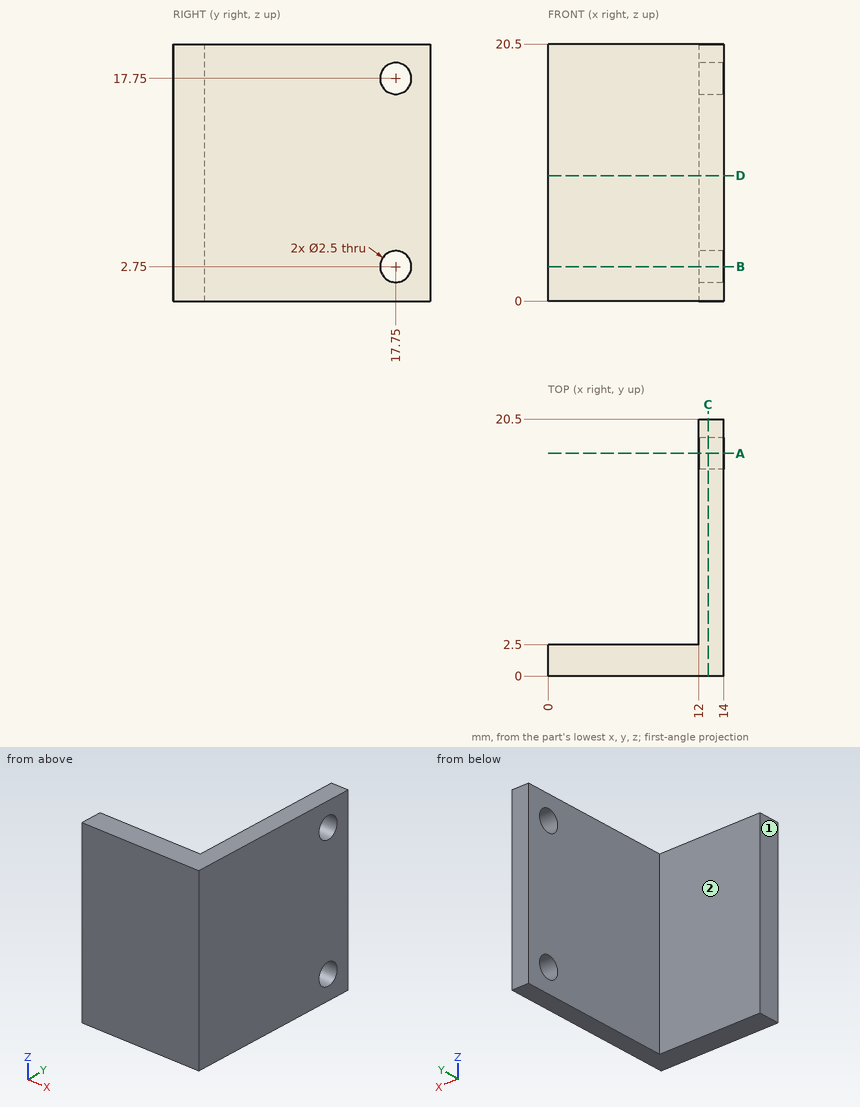
Answer from the drawing. Dimensions are ordinates in mm from the lowest x, y and z of the part. A direction names the side the tool comes from. Give positions to 0.01 mm unless a question says otherwise; leave off trailing zeros. Order: outer loops, then holes, each group sorted by start corner. A loop starts at its lowest first (then second) coordinate and runs counter-clockwise, first axis right, second up. Notation, with made-up numbers: (27.25, 24) -> (64.25, 24) arc R13 ccw to (64.25, 46) -> close; hole circle Ø7 at (61, 80). An arc over 180 degrees is marked (long way). One line per item, written item: value. Start each with the question number.
(1) The part is cut by section C-C (x = 12.75). Determine the outline of the cut face in (y, z), and give its area (3 significant figures).
(2) The part is cut by section B-B (z = 2.75). Determine the outline of the cut face in (x, y).
(3) Straight lines are drawn through the part: L1, parallel to Y at x = 12.55, z = 2.75; L2, parallel to Y at x = 2, z = 11.75; L3, parallel to X at y = 6.75, z = 9. For each, find the intervals that lie inside material, in ascending order.
(4) The part is cut by section D-D (z = 10). Determine the outline of the cut face in (x, y), and give its area (3 significant figures).
(5) A tool of negligible diameter and unlimited length cuts with its end or side. For the marked faces 1 and 2, from which of +Z, -Z, +X, -X, +Y, -Y can it reach the whole face along a straight path? Write none if from no direction.
(6) The part is cut by section A-A (y = 17.75). Determine the outline of the cut face in (x, z).
(7) Flat-ended cylindrical pins translate along their axes: P1, Ø4, axis at x = 11.5, y = 16.5, coming from the +Z side; P2, Ø1.5, axis at x = 2, z = 9.5, coming from the +Y side; P3, Ø8, axis at y = 13.5, z = 8.5, coming from the -X side; P4, Ø2, axis at y = 17.75, z = 2.75, coming from the +X side. Find the tip coordinate at first contact, or state that the pin passes through.
Taken from the geometry:
1. outline: (0, 0) -> (20.5, 0) -> (20.5, 20.5) -> (0, 20.5) -> close; hole circle Ø2.5 at (17.75, 2.75); hole circle Ø2.5 at (17.75, 17.75)
1. area: 410 mm^2
2. outline: (0, 0) -> (14, 0) -> (14, 16.5) -> (12, 16.5) -> (12, 2.5) -> (0, 2.5) -> close; (12, 19) -> (14, 19) -> (14, 20.5) -> (12, 20.5) -> close
3. L1: 0 to 16.5, 19 to 20.5
3. L2: 0 to 2.5
3. L3: 12 to 14
4. outline: (0, 0) -> (14, 0) -> (14, 20.5) -> (12, 20.5) -> (12, 2.5) -> (0, 2.5) -> close
4. area: 71.0 mm^2
5. face 1: +Z, -Z, -X, +Y, -Y
5. face 2: +Z, -Z, -X, +Y
6. outline: (12, 0) -> (14, 0) -> (14, 1.5) -> (12, 1.5) -> close; (12, 4) -> (14, 4) -> (14, 16.5) -> (12, 16.5) -> close; (12, 19) -> (14, 19) -> (14, 20.5) -> (12, 20.5) -> close
7. P1: z = 20.5
7. P2: y = 2.5
7. P3: x = 12
7. P4: through
